```python
from build123d import *

# Parameters (mm, degrees)
SKICA1_R                = 7
P_IDAT_VYSUNUT_M1_DEPTH = 3
SKICA2_R                = 5
P_IDAT_VYSUNUT_M2_DEPTH = 20
ZAOBLIT1_R              = 1


with BuildPart() as part:
    # Skica1 → Přidat vysunutím1 (new body)
    with BuildSketch(Plane.XY):
        Circle(SKICA1_R)
    extrude(amount=P_IDAT_VYSUNUT_M1_DEPTH)

    # Skica2 → Přidat vysunutím2 (add)
    with BuildSketch(Plane(origin=(0, 0, 0), x_dir=(-1, 0, 0), z_dir=(0, 0, -1))):
        Circle(SKICA2_R)
    extrude(amount=P_IDAT_VYSUNUT_M2_DEPTH)

    # Zaoblit1
    zaoblit1_edges = [part.edges().sort_by_distance(p)[0] for p in [
        (-7, 0, 3),
        (5, 0, -20),
    ]]
    fillet(zaoblit1_edges, radius=ZAOBLIT1_R)


solid = part.part
```
Could you check a few things on this model? Use its own coordinates, in mm. A direction names the side the tool comes from. Coordinates: 2 decimals unless noted, no trailing zeros. Loops run counter-clockwise (first coordinate to the right, second up) from the corner with the lowest first, then second, coordinate; pieces in that order, holes last.
1) Imagine slicing it at C-C (z = -17.5). List the corners of the cut face in (x, y) for me.
Reported:
outline: circle Ø10 at (0, 0)
2) Will these pins go through, and if not, where does the flat tip stop? pin 1 Ø1 at (x, z) = (4.5, -10) entering from -Y; pin 2 Ø4 at (x, z) = (1, -1.5) entering from -Y; pin 3 Ø1 at (x, y) = (-2, 4.5) entering from -Z; pin 4 Ø3 at (x, z) = (-2.5, -14.5) entering from -Y.
Reported:
pin 1: stops at y = -3
pin 2: stops at y = -7
pin 3: stops at z = -19.91
pin 4: stops at y = -4.9
3) Which directions (+Z, -Z, +X, -X, +Y, -Y) give clear straight access to the entire face, cutting with the end or side of a thin tool? Please do faces 1 (the face through (-2, 5, 0)), 2 (the face through (0, 0, -20)).
Reported:
face 1: -Z
face 2: -Z, +X, -X, +Y, -Y
4) Imagine slicing it at A-A (x = 0). List the corners of the cut face in (y, z) for me, and give its area (3 significant figures).
Reported:
outline: (-7, 0) - (-5, 0) - (-5, -19) arc R1 ccw to (-4, -20) - (4, -20) arc R1 ccw to (5, -19) - (5, 0) - (7, 0) - (7, 2) arc R1 ccw to (6, 3) - (-6, 3) arc R1 ccw to (-7, 2) - close
area: 241 mm2
5) Please list where these lines run through material, in increasing order: line 1 along Y through (x, z) = (-3, -5.5); line 2 along Z through (x, y) = (-5.25, -2.25); line 3 along Y through (x, z) = (4, 0.25).
Reported:
line 1: y = -4 to 4
line 2: z = 0 to 3
line 3: y = -5.74 to 5.74
